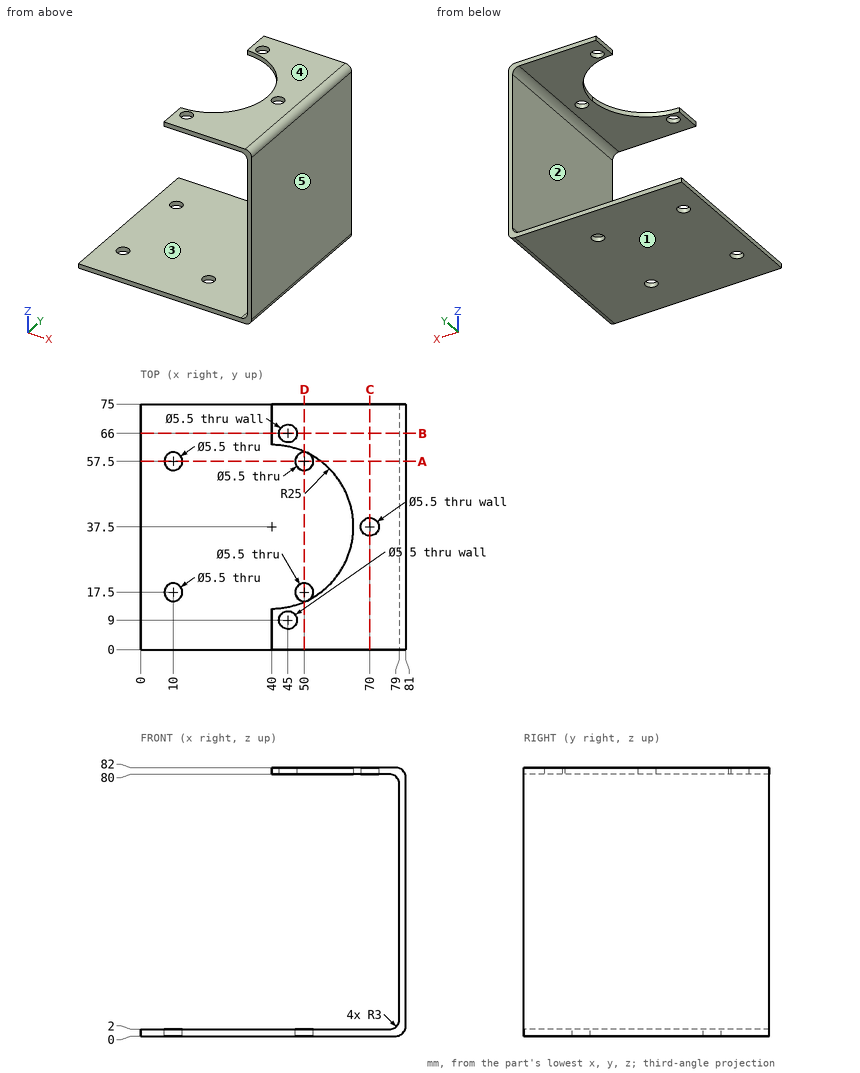
The figure shows three views and two pictorial views of one solid part (mm, origin at its lowest corner). Answer the questions. A direction names the side the tool comes from. Give positions to 0.01 mm unless a question says otherwise; leave off trailing zeros. Write each loop counter-clockwise with the first axis right and the second up, starting at its lowest first coordinate (ties: lowest second). Pieces come first, ordered by that corner, then holes. Notation, with made-up numbers: (-26.5, 32) -> (0.5, 32) arc R22 cw to (0.5, 40) -> close; hole circle Ø9 at (-10.75, -23.5). An arc over 180 degrees is marked (long way). Answer as a JSON object with one key per item and string values.
1) Flat-ended cylindrical pins translate along their axes: pin 1 Ø12 at (y, z) = (44, 63.5) entering from -X; pin 2 Ø6.5 at (x, y) = (50, 57.5) entering from +Z; pin 3 Ø8 at (x, y) = (27, 65) entering from +Z; pin 4 Ø1.6 at (y, z) = (4, 81) entering from -X. Find the tip coordinate at first contact, or state that the pin passes through.
Findings below:
{"pin 1": "stops at x = 79", "pin 2": "stops at z = 82", "pin 3": "stops at z = 2", "pin 4": "stops at x = 40"}
2) Section C-C on x = 70 is taken. Write down the section's boundary in (y, z), then the cut area to 3 significant figures.
Findings below:
{"outline": "(0, 0) -> (75, 0) -> (75, 2) -> (0, 2) -> close; (0, 80) -> (34.75, 80) -> (34.75, 82) -> (0, 82) -> close; (40.25, 80) -> (75, 80) -> (75, 82) -> (40.25, 82) -> close", "area": "289 mm^2"}
3) Section A-A on y = 57.5 is taken. Write down the section's boundary in (x, z).
Findings below:
{"outline": "(0, 0) -> (7.25, 0) -> (7.25, 2) -> (0, 2) -> close; (12.75, 0) -> (47.25, 0) -> (47.25, 2) -> (12.75, 2) -> close; (52.75, 0) -> (78, 0) arc R3 ccw to (81, 3) -> (81, 79) arc R3 ccw to (78, 82) -> (55, 82) -> (55, 80) -> (76, 80) arc R3 cw to (79, 77) -> (79, 5) arc R3 cw to (76, 2) -> (52.75, 2) -> close"}
4) Section D-D on x = 50 is taken. Write down the section's boundary in (y, z).
Findings below:
{"outline": "(0, 0) -> (14.75, 0) -> (14.75, 2) -> (0, 2) -> close; (0, 80) -> (14.59, 80) -> (14.59, 82) -> (0, 82) -> close; (20.25, 0) -> (54.75, 0) -> (54.75, 2) -> (20.25, 2) -> close; (60.25, 0) -> (75, 0) -> (75, 2) -> (60.25, 2) -> close; (60.41, 80) -> (75, 80) -> (75, 82) -> (60.41, 82) -> close"}
5) Straight lines are drawn through the part: probe 1 along Y at (x, z) = (50, 1.2); probe 2 along Z at (x, y) = (43.5, 4.5); probe 3 along Z at (x, y) = (4.5, 4). For each, find the intervals that lie inside material, in ascending order. Write a range as from..to.
Findings below:
{"probe 1": "y = 0..14.75, 20.25..54.75, 60.25..75", "probe 2": "z = 0..2, 80..82", "probe 3": "z = 0..2"}
6) A tool of negligible diameter and unlimited length cuts with its end or side. For the marked faces 1 and 2, from which of +Z, -Z, +X, -X, +Y, -Y can it reach the whole face along a straight path? Write none if from no direction.
Findings below:
{"face 1": "-Z, +X, -X, +Y, -Y", "face 2": "-X, +Y, -Y"}
7) For a pull along Z with two mould halves and no side action, classify the marked faces 3, 4 and 5 as pulls with the +Z half, pulls with the -Z half, needs draft (parallel to the pull), parting line crosses it, or undercut.
Findings below:
{"face 3": "undercut", "face 4": "pulls with the +Z half", "face 5": "needs draft"}
8) Section B-B on y = 66 is taken. Write down the section's boundary in (x, z), then the cut area to 3 significant figures.
Findings below:
{"outline": "(0, 0) -> (78, 0) arc R3 ccw to (81, 3) -> (81, 79) arc R3 ccw to (78, 82) -> (47.75, 82) -> (47.75, 80) -> (76, 80) arc R3 cw to (79, 77) -> (79, 5) arc R3 cw to (76, 2) -> (0, 2) -> close; (40, 80) -> (42.25, 80) -> (42.25, 82) -> (40, 82) -> close", "area": "389 mm^2"}
